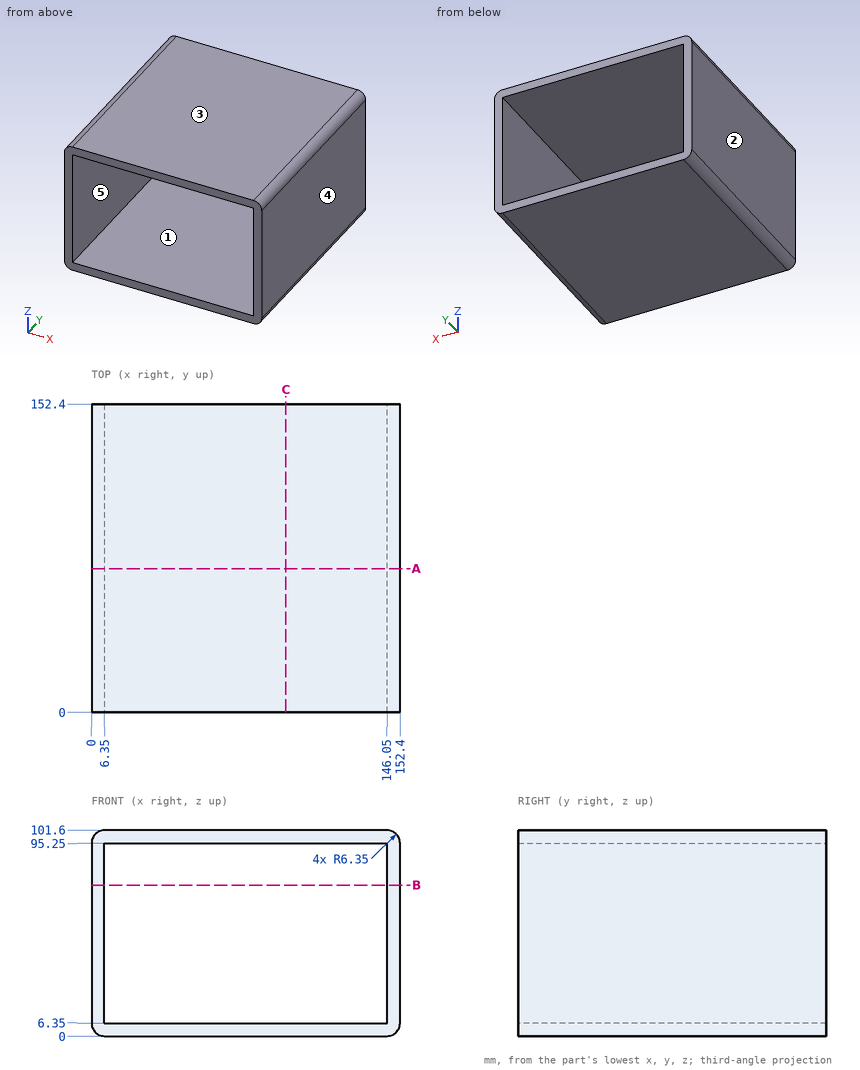
Job drawing, mm, ordinate dimensions from the low corner. One solid piece. A direction names the side the tool comes from. Give positions to 0.01 mm unless a question says otherwise; leave off trailing zeros. Loops run counter-clockwise (first coordinate to the right, second up) from the corner with the lowest first, then second, coordinate; pieces in that order, holes last. Notation, with made-up numbers: M -0.5,64.25 L 44.5,64.25 A21 ccw 44.5,80.25 Z; hole C -30.5,60.5 d1. An arc over 180 degrees is marked long. Answer in a Markdown table with one row per item. Add a question column.
Item 1: Probe probe 1 along X at (y, z) = (92.5, 37); probe 2 along Z at (x, y) = (120.5, 52); probe 3 along X at (y, z) = (116, 5). List the from-to ranges inside material, lowest first.
Item 2: Band-saw the part on B-B on z = 74.5. Give the cut face in (x, y), then the cut area to 3 significant figures.
Item 3: Tool access for the marked faces 4 and 5: list every direction of +Z, -Z, +X, -X, +Y, -Y with a clear straight run to the whole face (end or side of a thin tool).
Item 4: Mould opens along X. For the marked faces 1, 2 and 3 say: +X half, -X half, draft (parallel to the pull), parting line (faces both ways), or undercut.
Item 5: Band-saw the part on C-C on x = 96. Give the cut face in (y, z).
Item 6: Band-saw the part on A-A on y = 71. Give the cut face in (x, z).
Reply:
| question | item | result |
|---|---|---|
| 1 | probe 1 | x = 0 to 6.35, 146.05 to 152.4 |
| 1 | probe 2 | z = 0 to 6.35, 95.25 to 101.6 |
| 1 | probe 3 | x = 0.15 to 152.25 |
| 2 | outline | M 0,0 L 6.35,0 L 6.35,152.4 L 0,152.4 Z; M 146.05,0 L 152.4,0 L 152.4,152.4 L 146.05,152.4 Z |
| 2 | area | 1,940 mm^2 |
| 3 | face 4 | +Z, -Z, +X, +Y, -Y |
| 3 | face 5 | +Y, -Y |
| 4 | face 1 | undercut |
| 4 | face 2 | -X half |
| 4 | face 3 | draft |
| 5 | outline | M 0,0 L 152.4,0 L 152.4,6.35 L 0,6.35 Z; M 0,95.25 L 152.4,95.25 L 152.4,101.6 L 0,101.6 Z |
| 6 | outline | M 0,6.35 A6.35 ccw 6.35,0 L 146.05,0 A6.35 ccw 152.4,6.35 L 152.4,95.25 A6.35 ccw 146.05,101.6 L 6.35,101.6 A6.35 ccw 0,95.25 Z; hole M 6.35,6.35 L 146.05,6.35 L 146.05,95.25 L 6.35,95.25 Z |
